from build123d import *

# Parameters (mm, degrees)
F0_R     = 14.024991
F0_R_2   = 12.524994
F1_DEPTH = 28.049982
F2_R     = 14.024991
F2_R_2   = 12.524994
F3_DEPTH = 28.049982
F4_DEPTH = 25.4


with BuildPart() as f1:
    # F0 (on Right) → F1 (new body, symmetric)
    with BuildSketch(Plane.YZ):
        Circle(F0_R)
        Circle(F0_R_2, mode=Mode.SUBTRACT)
    extrude(amount=F1_DEPTH, both=True)

    # F2 (on Top) → F3 (join)
    with BuildSketch(Plane.XY):
        Circle(F2_R)
        Circle(F2_R_2, mode=Mode.SUBTRACT)
    extrude(amount=F3_DEPTH)

    # F0 (on Right) → F4 (cut, symmetric)
    with BuildSketch(Plane.YZ):
        Circle(F0_R_2)
    extrude(amount=F4_DEPTH, both=True, mode=Mode.SUBTRACT)


solid = f1.part
Input: part model. Units: mm. Frame: model coordinates. A direction names the side the tool comes from. Give positions to 0.01 mm unless a question says otherwise; leave off trailing zeros. Write each loop counter-clockwise with the first axis right and the second up, starting at its lowest first coordinate (ties: lowest second). Pieces come first, ordered by that corner, then holes.
Q1. Set-up query: faces 5 (the face through (-0.393, -2.715, -12.227)), 6 (the face through (13.38, 4.21, 16.95)). Return all of +Z, -Z, +X, -X, +Y, -Y with unobstructed straight access to the full face (end or side cutting, diameter ignored); none if empty.
Q2. Material intervals for probe 1 along Z at (x, y) = (4, 0) (3 decimals); probe 2 along Y at (x, z) = (-22, -1.5), sorted ascending.
Q3. First-contact query: P1, Ø1, axis at y = 9.5, z = 15, coming from the -X side; P2, Ø4, axis at y = -2, z = 21, coming from the +X side (3 decimals); P3, Ø15, axis at y = 0, z = 0, coming from the +X side; P4, Ø6, axis at x = -7, y = -5, coming from the -Z side. Flat tips, straight axial feed; report the tip coordinate or a pass-through.
Q4. Section C-C, the plane z = -2. Output: boundary loops of the cut face in (x, y).
Q5. Section B-B, the plane x = 0. Output: boundary loops of the cut face in (y, z) (3 decimals), plus the area to 4 significant figures.
Q6. Pull-direction query (Y, two-part tool) for faces 1 (the face through (-12.513, 0.551, 19.444)), 2 (the face through (0.163, 0.217, 14.023)), 3 (the face through (0.4, -3, -13.7)), 4 (the face through (-28.05, 0, 13)); classes: pulls with the +Y half, pulls with the -Y half, needs draft (parallel to the pull), parting line crosses it, or undercut.
Q7. Section A-A, the plane y = 0. Output: boundary loops of the cut face in (x, z) (3 decimals), plus the area to 3 significant figures.
Q8. Section D-D, the plane y = 7.25. Output: boundary loops of the cut face in (x, z), plus the area to 3 significant figures.
Filled in:
1. face 5: +X, -X
1. face 6: +Z
2. probe 1: z = -14.025 to -12.525, 12.525 to 14.025
2. probe 2: y = -13.94 to -12.43, 12.43 to 13.94
3. P1: stops at x = -10.76
3. P2: stops at x = 14.025
3. P3: passes through
3. P4: stops at z = -13.88
4. outline: (-28.05, -13.88) - (28.05, -13.88) - (28.05, -12.36) - (-28.05, -12.36) - close; (-28.05, 12.36) - (28.05, 12.36) - (28.05, 13.88) - (-28.05, 13.88) - close
5. outline: (-14.025, 0) arc R14.025 ccw to (14.025, 0) - (14.025, 28.05) - (12.525, 28.05) - (12.525, 6.311) arc R14.025 ccw to (-12.525, 6.311) - (-12.525, 28.05) - (-14.025, 28.05) - close; hole circle Ø25.05 at (0, 0)
5. area: 196.5 mm2
6. face 1: undercut
6. face 2: undercut
6. face 3: parting line crosses it
6. face 4: needs draft
7. outline: (-28.05, -14.025) - (28.05, -14.025) - (28.05, -12.525) - (-28.05, -12.525) - close; (-28.05, 12.525) - (28.05, 12.525) - (28.05, 14.025) - (14.025, 14.025) - (14.025, 28.05) - (12.525, 28.05) - (12.525, 14.025) - (-12.525, 14.025) - (-12.525, 28.05) - (-14.025, 28.05) - (-14.025, 14.025) - (-28.05, 14.025) - close
7. area: 210 mm2
8. outline: (-28.05, -12.01) - (28.05, -12.01) - (28.05, -10.21) - (-28.05, -10.21) - close; (-28.05, 10.21) - (28.05, 10.21) - (28.05, 12.01) - (12.01, 12.01) - (12.01, 28.05) - (10.21, 28.05) - (10.21, 12.01) - (-10.21, 12.01) - (-10.21, 28.05) - (-12.01, 28.05) - (-12.01, 12.01) - (-28.05, 12.01) - close
8. area: 259 mm2
